Part print with two shaded views. Sizes in mm from the minimum x, y, z corner. A direction names the side the tool comes from. Round coordinates to 2 decimals unless told otherwise and drop trailing zeros. Order: outer loops, then holes, each group sorted by start corner. A loop starts at its lowest first (then second) coordinate and runs counter-clockwise, first axis right, second up. Notation, with made-up numbers: (1.5, 17.5) - (23.5, 17.5) arc R10 ccw to (23.5, 29.5) - close; hole circle Ø1 at (-16.5, 48). An arc over 180 degrees is marked (long way). Write item = value, one per line.
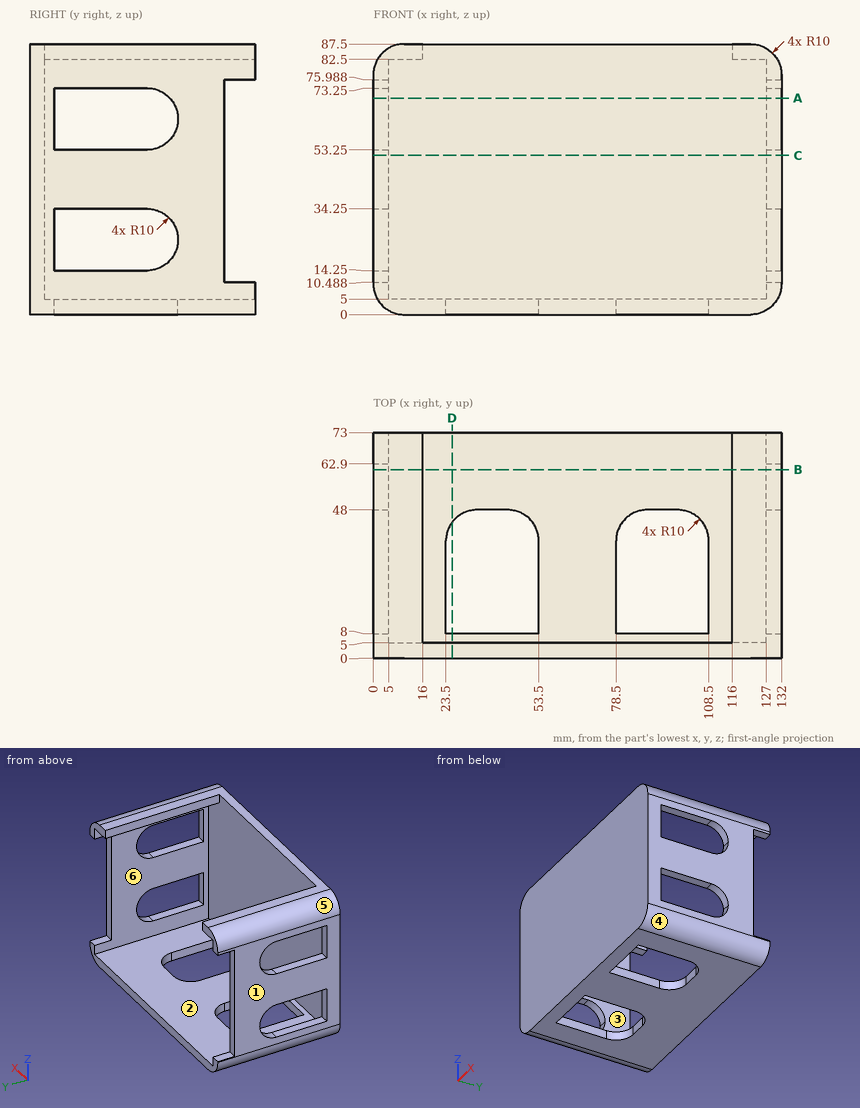
1) Flat gauge pins, fed straight in: pin 1 Ø2.5 at (x, y) = (130, 19) entering from -Z; pin 2 Ø4 at (x, z) = (129, 63.5) entering from +Y; pin 3 Ø4 at (y, z) = (36, 86) entering from -X. Where does each tip first touch, or does it go through?
Conclusion:
pin_1 = 2.62
pin_2 = 62.9
pin_3 = 2.4
2) Wall check: line 1 along X through (y, z) = (51, 63.5); line 2 along Z through (x, y) = (10, 18.5); line 3 along Y through (x, z) = (10, 19.5). Give the ranges that are in metal, low to high.
Conclusion:
line_1 = 0 to 5, 127 to 132
line_2 = 0 to 5, 82.5 to 87.5
line_3 = 0 to 5
3) Cut at B-B (y = 61). Write the cut outline in (x, z).
Conclusion:
outline = (0, 10) arc R10 ccw to (10, 0) - (122, 0) arc R10 ccw to (132, 10) - (132, 77.5) arc R10 ccw to (122, 87.5) - (116, 87.5) - (116, 82.5) - (127, 82.5) - (127, 5) - (5, 5) - (5, 82.5) - (16, 82.5) - (16, 87.5) - (10, 87.5) arc R10 ccw to (0, 77.5) - close
4) Cut at D-D (x = 25.5). Write the cut outline in (y, z).
Conclusion:
outline = (0, 0) - (8, 0) - (8, 5) - (5, 5) - (5, 87.5) - (0, 87.5) - close; (44, 0) - (73, 0) - (73, 5) - (44, 5) - close
5) Cut at C-C (z = 51.5). Write the cut outline in (x, y), and give its area (3 significant figures).
Conclusion:
outline = (0, 0) - (132, 0) - (132, 62.9) - (127, 62.9) - (127, 5) - (5, 5) - (5, 62.9) - (0, 62.9) - close
area = 1,240 mm^2
6) 3-axis set-ups, long thin cutter, end or side, ignore diameter. For the marked faces 1 and 2: which of +Z, -Z, +X, -X, +Y, -Y reach the whole face in a straight line?
Conclusion:
face_1 = +Z, -Z, -X, +Y, -Y
face_2 = +Y
7) Mould opens along X. For the marked faces 3, 4, 5 and 6 say: +X half, -X half, draft (parallel to the pull), parting line (faces both ways), or undercut.
Conclusion:
face_3 = undercut
face_4 = +X half
face_5 = -X half
face_6 = undercut
8) Cut at A-A (z = 70). Write the cut outline in (x, y).
Conclusion:
outline = (0, 0) - (132, 0) - (132, 8) - (127, 8) - (127, 5) - (5, 5) - (5, 8) - (0, 8) - close; (0, 45.38) - (5, 45.38) - (5, 62.9) - (0, 62.9) - close; (127, 45.38) - (132, 45.38) - (132, 62.9) - (127, 62.9) - close
